Verification items for the finished model (mm, model axes). Give positions to 0.01 mm unless a question says otherwise; leave off trailing zeros. Order: outer loops, then holes, each group sorted by start corner. A loop starts at its lowest first (then second) coordinate and runs counter-clockwise, first axis right, second up.
from build123d import *

# Parameters (mm, degrees)
SKETCH_W        = 150
SKETCH_H        = 120
PAD_DEPTH       = 2
SKETCH001_W     = 90
SKETCH001_H     = 65
POCKET_DEPTH    = 2
SKETCH002_R     = 9
POCKET001_DEPTH = 2
SKETCH003_R     = 4.5
POCKET002_DEPTH = 2
POCKET003_DEPTH = 2
POCKET004_DEPTH = 2
POCKET005_DEPTH = 2
POCKET006_DEPTH = 2
POCKET007_DEPTH = 2
POCKET008_DEPTH = 2
FILLET_R        = 1.9


with BuildPart() as part:
    # Sketch → Pad (new body)
    with BuildSketch(Plane.XY):
        with Locations((75, 60)):
            Rectangle(SKETCH_W, SKETCH_H)
    extrude(amount=PAD_DEPTH)

    # Sketch001 → Pocket (cut)
    with BuildSketch(Plane.XY):
        with Locations((55, 77.5)):
            Rectangle(SKETCH001_W, SKETCH001_H)
    extrude(amount=POCKET_DEPTH, mode=Mode.SUBTRACT)

    # Sketch002 → Pocket001 (cut)
    with BuildSketch(Plane.XY):
        with Locations((125, 75)):
            Circle(SKETCH002_R)
    extrude(amount=POCKET001_DEPTH, mode=Mode.SUBTRACT)

    # Sketch003 → Pocket002 (cut)
    with BuildSketch(Plane.XY):
        with Locations((125, 50)):
            Circle(SKETCH003_R)
    extrude(amount=POCKET002_DEPTH, mode=Mode.SUBTRACT)

    # Sketch004 → Pocket003 (cut)
    with BuildSketch(Plane.XY):
        with BuildLine():
            ThreePointArc((21, 32.5), (20, 33.5), (19, 32.5))
            Line((19, 32.5), (19, 12.5))
            ThreePointArc((19, 12.5), (20, 11.5), (21, 12.5))
            Line((21, 32.5), (21, 12.5))
        make_face()
    extrude(amount=POCKET003_DEPTH, mode=Mode.SUBTRACT)

    # Sketch006 → Pocket004 (cut)
    with BuildSketch(Plane.XY):
        with BuildLine():
            ThreePointArc((26, 32.5), (25, 33.5), (24, 32.5))
            Line((24, 32.5), (24, 12.5))
            ThreePointArc((24, 12.5), (25, 11.5), (26, 12.5))
            Line((26, 32.5), (26, 12.5))
        make_face()
    extrude(amount=POCKET004_DEPTH, mode=Mode.SUBTRACT)

    # Sketch008 → Pocket005 (cut)
    with BuildSketch(Plane.XY):
        with BuildLine():
            ThreePointArc((31, 32.5), (30, 33.5), (29, 32.5))
            Line((29, 32.5), (29, 12.5))
            ThreePointArc((29, 12.5), (30, 11.5), (31, 12.5))
            Line((31, 32.5), (31, 12.5))
        make_face()
    extrude(amount=POCKET005_DEPTH, mode=Mode.SUBTRACT)

    # Sketch009 → Pocket006 (cut)
    with BuildSketch(Plane.XY):
        with BuildLine():
            ThreePointArc((81, 32.5), (80, 33.5), (79, 32.5))
            Line((79, 32.5), (79, 12.5))
            ThreePointArc((79, 12.5), (80, 11.5), (81, 12.5))
            Line((81, 32.5), (81, 12.5))
        make_face()
    extrude(amount=POCKET006_DEPTH, mode=Mode.SUBTRACT)

    # Sketch010 → Pocket007 (cut)
    with BuildSketch(Plane.XY):
        with BuildLine():
            ThreePointArc((86, 32.5), (85, 33.5), (84, 32.5))
            Line((84, 32.5), (84, 12.5))
            ThreePointArc((84, 12.5), (85, 11.5), (86, 12.5))
            Line((86, 32.5), (86, 12.5))
        make_face()
    extrude(amount=POCKET007_DEPTH, mode=Mode.SUBTRACT)

    # Sketch011 → Pocket008 (cut)
    with BuildSketch(Plane.XY):
        with BuildLine():
            ThreePointArc((91, 32.5), (90, 33.5), (89, 32.5))
            Line((89, 32.5), (89, 12.5))
            ThreePointArc((89, 12.5), (90, 11.5), (91, 12.5))
            Line((91, 32.5), (91, 12.5))
        make_face()
    extrude(amount=POCKET008_DEPTH, mode=Mode.SUBTRACT)

    # Fillet
    fillet_edges = [part.edges().sort_by_distance(p)[0] for p in [
        (0, 60, 2),
        (75, 0, 2),
        (0, 0, 1),
        (0, 120, 1),
        (75, 120, 2),
        (150, 60, 2),
        (150, 0, 1),
        (150, 120, 1),
    ]]
    fillet(fillet_edges, radius=FILLET_R)


solid = part.part
(1) Go/stop test with flat-tipped pins: pin 1 (0.6 mm diameter, centred on y = 19, z = 1, fed in from -X); pin 2 (0.6 mm diameter, centred on y = 25, z = 1.5, fed in from -X); pin 3 (0.6 mm diameter, centred on x = 51, z = 1, fed in from -Y). Record where each tip stops, or that it passes through.
Solved:
pin 1: stops at x = 0.1
pin 2: stops at x = 0.35
pin 3: stops at y = 0.1
(2) Section check C-C, the plane y = 50. Enter the section's corners in (x, z).
Solved:
outline: (0, 0) - (10, 0) - (10, 2) - (1.9, 2) arc R1.9 ccw to (0, 0.1) - close; (100, 0) - (120.5, 0) - (120.5, 2) - (100, 2) - close; (129.5, 0) - (150, 0) - (150, 0.1) arc R1.9 ccw to (148.1, 2) - (129.5, 2) - close
(3) Release check for a two-part mould opening along X. For faces 1 (the flat face through (74, 34, 0)), 2 (the cylindrical face through (129.153, 67.015, 0.986)) record: pulls with the +X half, pulls with the -X half, needs draft (parallel to the pull), parting line crosses it, or undercut.
Solved:
face 1: needs draft
face 2: undercut
(4) Section check A-A, the plane y = 87.5. Enter the section's corners in (x, z).
Solved:
outline: (0, 0) - (10, 0) - (10, 2) - (1.9, 2) arc R1.9 ccw to (0, 0.1) - close; (100, 0) - (150, 0) - (150, 0.1) arc R1.9 ccw to (148.1, 2) - (100, 2) - close
(5) Scan lines: line 1 (Y direction, x = 125, z = 0.9); line 2 (Y direction, x = 125, z = 0.6); line 3 (Y direction, x = 93, z = 0.4). Record each from-to range of solid material in increasing order.
Solved:
line 1: y = 0.18 to 45.5, 54.5 to 66, 84 to 119.82
line 2: y = 0.07 to 45.5, 54.5 to 66, 84 to 119.93
line 3: y = 0.02 to 45, 110 to 119.98
(6) Section check D-D, the plane x = 124.5. Enter the section's corners in (y, z).
Solved:
outline: (0, 0) - (45.53, 0) - (45.53, 2) - (1.9, 2) arc R1.9 ccw to (0, 0.1) - close; (54.47, 0) - (66.01, 0) - (66.01, 2) - (54.47, 2) - close; (83.99, 0) - (120, 0) - (120, 0.1) arc R1.9 ccw to (118.1, 2) - (83.99, 2) - close
(7) Section check B-B, the plane x = 74.5. Enter the section's corners in (y, z).
Solved:
outline: (0, 0) - (45, 0) - (45, 2) - (1.9, 2) arc R1.9 ccw to (0, 0.1) - close; (110, 0) - (120, 0) - (120, 0.1) arc R1.9 ccw to (118.1, 2) - (110, 2) - close
